from build123d import *

# Parameters (mm, degrees)
F0_R     = 2.5
F1_DEPTH = 5


with BuildPart() as f1:
    # F0 (on Front) → F1 (new body)
    with BuildSketch(Plane.XZ):
        with BuildLine():
            Line((0, 4), (-7.5, 4))
            ThreePointArc((-7.5, 4), (-11.5, 0), (-7.5, -4))
            Line((-7.5, -4), (0, -4))
            Line((0, -4), (0, 4))
        make_face()
        with Locations((-7.5, 0)):
            Circle(F0_R, mode=Mode.SUBTRACT)
        with BuildLine():
            Line((7.5, 4), (0, 4))
            Line((0, 4), (0, -4))
            Line((0, -4), (7.5, -4))
            ThreePointArc((7.5, -4), (11.5, 0), (7.5, 4))
        make_face()
        with Locations((7.5, 0)):
            Circle(F0_R, mode=Mode.SUBTRACT)
    extrude(amount=F1_DEPTH)


solid = f1.part
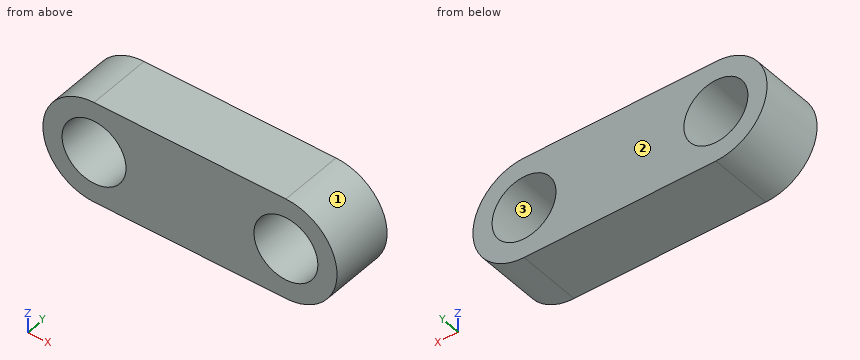
Geometry: final body of the model. Coordinates: model frame, mm. Face numbers are marked on the shaded views. Give positions to 0.01 mm unless a question says otherwise; leave off trailing zeros. Order: outer loops, then holes, each group sorted by start corner. A loop starts at its lowest first (then second) coordinate and runs counter-clockwise, first axis right, second up. Notation, with made-up numbers: (70.25, 68.5) -> (111.25, 68.5) arc R24 cw to (111.25, 99.5) -> close; hole circle Ø1 at (-2, 88.5). An arc over 180 degrees is marked (long way). Answer as a JSON object with one key per item and string values.
Q1. Section A-A (x = -5.5). Output: boundary loops of the cut face in (y, z).
Entries:
{"outline": "(-5, -4) -> (0, -4) -> (0, -1.5) -> (-5, -1.5) -> close; (-5, 1.5) -> (0, 1.5) -> (0, 4) -> (-5, 4) -> close"}
Q2. Section D-D (x = 7.25). Output: boundary loops of the cut face in (y, z), plus the area to 3 significant figures.
Entries:
{"outline": "(-5, -4) -> (0, -4) -> (0, -2.49) -> (-5, -2.49) -> close; (-5, 2.49) -> (0, 2.49) -> (0, 4) -> (-5, 4) -> close", "area": "15.1 mm^2"}
Q3. Material intervals for probe 1 along Z at (x, y) = (7.5, -3.6); probe 2 along X at (y, z) = (-2.9, -0.5); probe 3 along X at (y, z) = (-4.15, -1), sorted ascending.
Entries:
{"probe 1": "z = -4 to -2.5, 2.5 to 4", "probe 2": "x = -11.47 to -9.95, -5.05 to 5.05, 9.95 to 11.47", "probe 3": "x = -11.37 to -9.79, -5.21 to 5.21, 9.79 to 11.37"}
Q4. First-contact query: pin 1 (1.5 mm diameter, centred on x = -7, z = 0, fed in from +Y); pin 2 (1 mm diameter, centred on y = -3, z = -3, fed in from +X). Flat tips, straight axial feed; report the tip coordinate or a pass-through.
Entries:
{"pin 1": "passes through", "pin 2": "stops at x = 10.62"}
Q5. Section C-C (y = -0.35). Output: boundary loops of the cut face in (x, z).
Entries:
{"outline": "(-7.5, -4) -> (7.5, -4) arc R4 ccw to (7.5, 4) -> (-7.5, 4) arc R4 ccw to start; hole circle Ø5 at (-7.5, 0); hole circle Ø5 at (7.5, 0)"}
Q6. Section B-B (z = 0). Output: boundary loops of the cut face in (x, y), plus the area to 3 significant figures.
Entries:
{"outline": "(-11.5, -5) -> (-10, -5) -> (-10, 0) -> (-11.5, 0) -> close; (-5, -5) -> (5, -5) -> (5, 0) -> (-5, 0) -> close; (10, -5) -> (11.5, -5) -> (11.5, 0) -> (10, 0) -> close", "area": "65.0 mm^2"}
Q7. Draft query along Z for the marked faces 1, 2 and 3. Return one class per face: released by +Z, released by -Z, zero draft, split by the parting line, or undercut.
Entries:
{"face 1": "split by the parting line", "face 2": "zero draft", "face 3": "undercut"}
